For this review, use the dimensioned drawing (mm, ordinates from the lowest corner) and the shaded views. A direction names the side the tool comes from. Coordinates: 2 decimals unless noted, no trailing zeros. Loops run counter-clockwise (first coordinate to the right, second up) from the corner with the lowest first, then second, coordinate; pieces in that order, holes last. Notation, with made-up numbers: (46.5, 51) - (73.5, 51) arc R16 ccw to (73.5, 72) - close; hole circle Ø11 at (35.5, 4.25). An arc over 180 degrees is marked (long way). Use a Markdown table: item, result. Add a question column.
1) Clearance check with flat-ended pins moving along their axes: pin 1 (2 mm diameter, centred on x = 1.5, y = 1.5, fed in from -Z); pin 2 (5 mm diameter, centred on y = 5, z = 7, fed in from -X); pin 3 (1.5 mm diameter, centred on x = 3.5, z = 10.5, fed in from +Y). State where each tip first meets the part, or that it passes through.
2) Add section A-A, the plane x = 5. Give the boundary of the cut face in (y, z).
3) Add section D-D, the plane y = 1. Give the boundary of the cut face in (x, z), and give its area (3 significant figures).
4) To check wall thickness, follow L1, parallel to Z at x = 5.75, y = 2.5; L2, parallel to Z at x = 9.25, y = 5.75; L3, parallel to Y at x = 5, z = 12.75. State the ranges of each line that lie inside material, in increasing order. Write a range as [from, to].
5) For the marked faces 1, 2 and 3, list the 3-axis set-ups (+Z, -Z, +X, -X, +Y, -Y) from which the entire face can be reached by the end or side of a thin tool; tool diameter is ignored.
6) Add section C-C, the plane z = 5. Give the boundary of the cut face in (x, y).
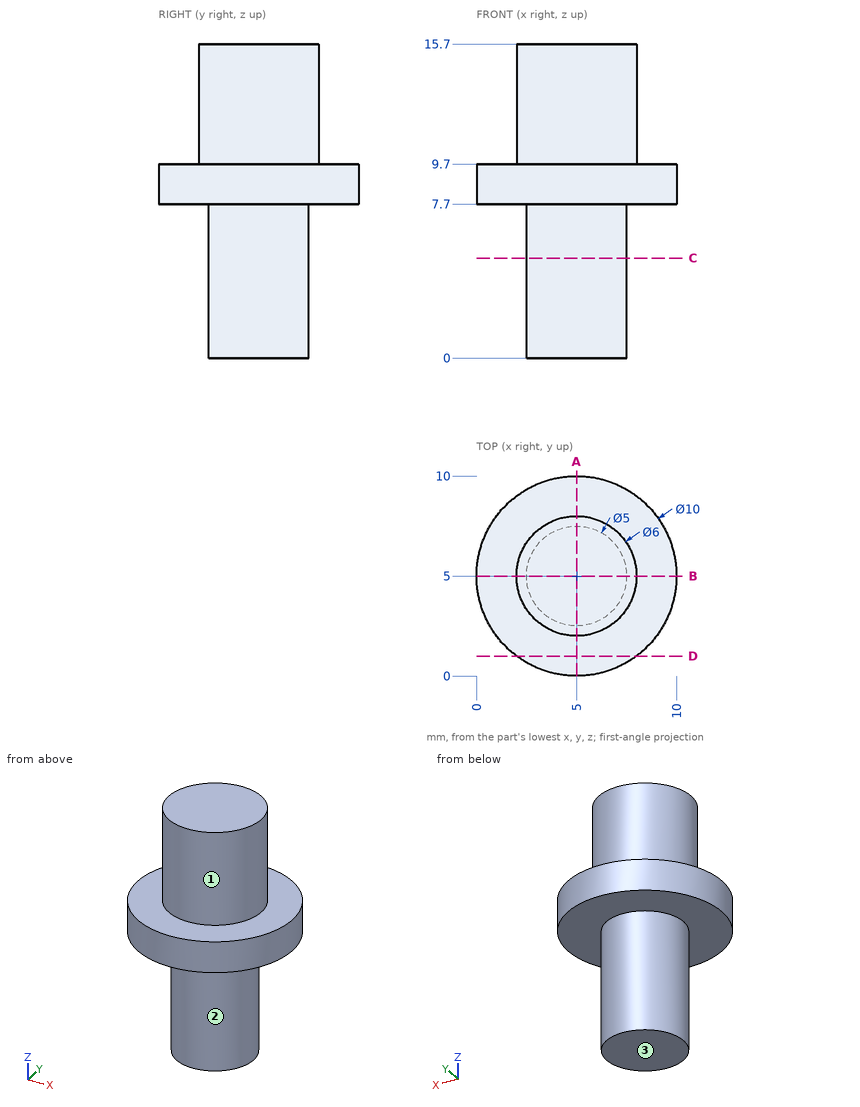
From the geometry:
| question | item | result |
|---|---|---|
| 1 | pin 1 | stops at z = 7.7 |
| 1 | pin 2 | stops at x = 0 |
| 1 | pin 3 | stops at y = 7.9 |
| 2 | outline | (0, 7.7) - (2.5, 7.7) - (2.5, 0) - (7.5, 0) - (7.5, 7.7) - (10, 7.7) - (10, 9.7) - (8, 9.7) - (8, 15.7) - (2, 15.7) - (2, 9.7) - (0, 9.7) - close |
| 3 | outline | (2, 7.7) - (8, 7.7) - (8, 9.7) - (2, 9.7) - close |
| 3 | area | 12.0 mm^2 |
| 4 | L1 | z = [7.7, 15.7] |
| 4 | L2 | z = [7.7, 9.7] |
| 4 | L3 | y = [2, 8] |
| 5 | face 1 | +Z |
| 5 | face 2 | -Z |
| 5 | face 3 | -Z, +X, -X, +Y, -Y |
| 6 | outline | circle Ø5 at (5, 5) |
